Geometry: final body of the model. Coordinates: model frame, mm. Round coordinates to 2 decimals unless told otherwise and drop trailing zeros. Write each loop counter-clockwise with the first axis right and the second up, starting at its lowest first coordinate (ties: lowest second). Pieces come first, ordered by that corner, then holes. Notation, with made-up numbers: M 71,67.5 L 122,67.5 A21 ccw 122,71.5 Z; hole C 42.25,20 d11. An arc over 180 degrees is marked long. Answer as CSV lines item,"result". Start each with the question number.
Q1. Section query A-A on z = 436.5. Output: boundary loops of the cut face in (x, y).
Q2. Section query B-B on y = 4.25. Output: boundary loops of the cut face in (x, z), and give its area (3 significant figures).
Q3. First-contact query: pin 1 (5 mm diameter, centred on y = 9, z = 466, fed in from +X); pin 2 (6 mm diameter, centred on y = 6, z = 106, fed in from +X); pin 3 (5 mm diameter, centred on y = 4, z = 319.5, fed in from +X). Flat tips, straight axial feed; report the tip coordinate or a pass-through.
Q4. Ray query, probe 1 along X at (y, z) = (3.75, 606); probe 2 along X at (y, z) = (4, 698); probe 3 along X at (y, z) = (9.75, 376). Return the intervals inside material, ascending.
```python
from build123d import *


with BuildPart() as part:
    # Varredura1: sweep along a path in Esboço2
    with BuildLine(Plane(origin=(0, 0, 0), x_dir=(1, 0, 0), z_dir=(0, 1, 0))) as varredura1_path:
        Line((0, 0), (0, -750))
    # Esboço1 → Varredura1 (sweep)
    with BuildSketch(Plane.XY):
        Polygon((0, 11.228855685), (8.980256121, 2.248599564), (6.731656557, 0), (0, 6.731656557), (-6.731656557, 0), (-8.980256121, 2.248599564), align=None)
    sweep(path=varredura1_path.line)


solid = part.part
```
Entries:
1,outline,"M -8.98,2.25 L -6.73,0 L 0,6.73 L 6.73,0 L 8.98,2.25 L 0,11.23 Z"
2,outline,"M -6.98,0 L -2.48,0 L -2.48,750 L -6.98,750 Z; M 2.48,0 L 6.98,0 L 6.98,750 L 2.48,750 Z"
2,area,"6,750 mm^2"
3,pin 1,"stops at x = 4.73"
3,pin 2,"stops at x = 8.23"
3,pin 3,"stops at x = 8.98"
4,probe 1,"x = -7.48 to -2.98, 2.98 to 7.48"
4,probe 2,"x = -7.23 to -2.73, 2.73 to 7.23"
4,probe 3,"x = -1.48 to 1.48"
